Can you work these out from the model? Positions are in its coordinate system, mm. Face numbers are marked on the shaded views. A direction names the side the tool comes from. Give positions to 0.01 mm unless a question says otherwise; leave off trailing zeros. Loops run counter-clockwise (first coordinate to the right, second up) from the corner with the lowest first, then second, coordinate; pieces in that order, holes last. Notation, with made-up numbers: M -12,-38 L -3,-38 A31 ccw -3,-12 Z; hole C -19,34 d4. An arc over 180 degrees is marked long. Answer as a JSON object with one key per item and string values.
```python
from build123d import *

# Parameters (mm, degrees)
EXTRUDE_THIN1_DEPTH = 5.5
FILLET1_R           = 5.5
SKETCH3_R           = 1
CUT_EXTRUDE1_DEPTH  = 23.726524062
SKETCH4_R           = 2.25
CUT_EXTRUDE2_DEPTH  = 2
SKETCH5_R           = 3
BOSS_EXTRUDE1_DEPTH = 10


with BuildPart() as part:
    # Sketch2 → Extrude-Thin1 (new, symmetric)
    with BuildSketch(Plane(origin=(0, 0, 0), x_dir=(0, 0, -1), z_dir=(1, 0, 0))):
        Polygon((0, 0), (-10, 0), (-19.396926208, -3.420201433), (-20.765006781, 0.33856905), (-10.705307923, 4), (0, 4), align=None)
    extrude(amount=EXTRUDE_THIN1_DEPTH, both=True)

    # Fillet1
    fillet1_edges = [part.edges().sort_by_distance(p)[0] for p in [
        (-5.5, 2, 0),
        (5.5, 2, 0),
    ]]
    fillet(fillet1_edges, radius=FILLET1_R - 0.0001)  # a hair under: the kernel refuses the full size

    # Sketch3 → Cut-Extrude1 (cut, through all)
    with BuildSketch(Plane(origin=(0, 4, 0), x_dir=(1, 0, 0), z_dir=(0, 1, 0))):
        with Locations(Location((0, -5.5, 0), (0, 0, 270))):
            Circle(SKETCH3_R)
    extrude(amount=-CUT_EXTRUDE1_DEPTH, mode=Mode.SUBTRACT)

    # Sketch4 → Cut-Extrude2 (cut)
    with BuildSketch(Plane.XZ):
        with Locations(Location((0, 5.5, 0), (0, 0, 270))):
            Circle(SKETCH4_R)
    extrude(amount=-CUT_EXTRUDE2_DEPTH, mode=Mode.SUBTRACT)

    # Sketch5 → Boss-Extrude1 (add)
    with BuildSketch(Plane(origin=(0, -6.634139482, 18.227148423), x_dir=(1, 0, 0), z_dir=(0, -0.34202014332567143, 0.9396926207859075))):
        with BuildLine():
            Line((5.5, 7.420201433), (5.5, 10.920201433))
            ThreePointArc((5.5, 10.920201433), (0, 16.420201433), (-5.5, 10.920201433))
            Line((-5.5, 10.920201433), (-5.5, 7.420201433))
            Line((-5.5, 7.420201433), (-5.5, 3.420201433))
            Line((-5.5, 3.420201433), (5.5, 3.420201433))
            Line((5.5, 3.420201433), (5.5, 7.420201433))
        make_face()
        with Locations(Location((0, 10.920201433, 0), (0, 0, 270))):
            Circle(SKETCH5_R, mode=Mode.SUBTRACT)
    extrude(amount=-BOSS_EXTRUDE1_DEPTH)


solid = part.part
```
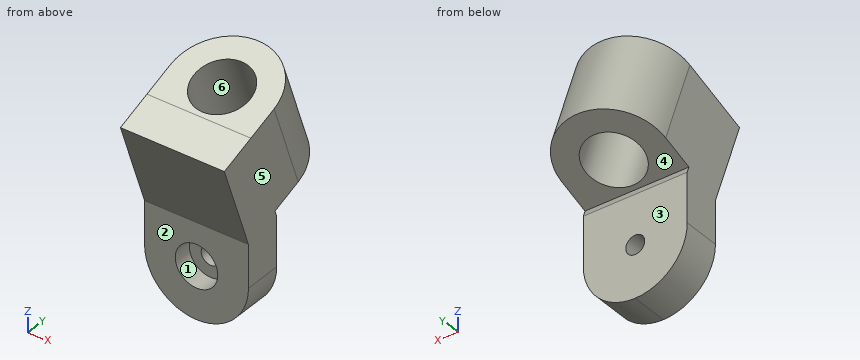
1) For the marked faces 1, 2 and 3, which set-ups out of +Z, -Z, +X, -X, +Y, -Y let a thin tool reach every point of the face, with its end or its side?
Answer list:
{"face 1": "-Y", "face 2": "-Z, +X, -X, -Y", "face 3": "-Z, +X, -X, +Y"}
2) Suppose I cut it at C-C, the plane x = 3.5. Write out the boundary of the cut face in (y, z) (3 decimals), and give its area (3 significant figures).
Answer list:
{"outline": "M -3.42,19.397 L 0,10 L 0,1.257 L 4,1.257 L 4,10.705 L 3.759,11.368 L 11.034,14.016 L 7.614,23.413 Z", "area": "155 mm^2"}
3) If we mould it in two halves opening along X, with no side actions, what happens to the marked faces 4, 5 and 6? For each: +X half, -X half, draft (parallel to the pull), parting line (faces both ways), or undercut.
Answer list:
{"face 4": "draft", "face 5": "+X half", "face 6": "undercut"}
4) Will these pins go through, and if not, where does the flat tip stop? pin 1 Ø3 at (x, z) = (0, 7.5) entering from +Y; pin 2 Ø1.5 at (x, y) = (4, 2.5) entering from +Z; pin 3 Ø3 at (x, z) = (0.5, 15) entering from -Y.
Answer list:
{"pin 1": "y = 4", "pin 2": "z = 21.82", "pin 3": "y = -2.37"}
5) Please list where these lines run through material, in increasing order: line 1 along X through (y, z) = (0.55, 5.5); line 2 along X through (y, z) = (2.9, 5.5); line 3 along Y through (x, z) = (0.25, 3.75). Write a range as from..to.
Answer list:
{"line 1": "-5.5..-2.25, 2.25..5.5", "line 2": "-5.5..-1, 1..5.5", "line 3": "2..4"}
6) Suppose I cut it at A-A, the plane x = -0.75. Write out the boundary of the cut face in (y, z) (3 decimals).
Answer list:
{"outline": "M -3.42,19.397 L 0,10 L 0,7.621 L 2,7.621 L 2,6.161 L 4,6.161 L 4,10.705 L 3.759,11.368 L 4.318,11.572 L 0.898,20.969 Z; M 0,0.051 L 4,0.051 L 4,4.839 L 2,4.839 L 2,3.379 L 0,3.379 Z; M 6.357,22.956 L 9.777,13.559 L 12.168,14.429 L 8.748,23.826 Z"}
7) Suppose I cut it at B-B, the plane z = 8.5. Write out the boundary of the cut face in (x, y).
Answer list:
{"outline": "M -5.5,0 L 5.5,0 L 5.5,4 L -5.5,4 Z"}
8) Suppose I cut it at D-D, the plane x = -4.5. Write out the boundary of the cut face in (y, z) (3 decimals), and give its area (3 significant figures).
Answer list:
{"outline": "M -3.42,19.397 L 0,10 L 0,2.338 L 4,2.338 L 4,10.705 L 3.759,11.368 L 10.019,13.647 L 6.599,23.044 Z", "area": "140 mm^2"}
